Read the model definition and answer for the solid it produces. Units are mm, in the model's axes. Coordinates: 2 decimals unless noted, no trailing zeros. Write each loop counter-clockwise with the first axis right and the second up, starting at its lowest first coordinate (ties: lowest second). Pieces come first, ordered by that corner, then holes. Notation, with made-up numbers: (-30, -32.75) -> (-4, -32.75) arc R25 ccw to (-4, -11.75) -> close; hole circle Ø9 at (67, -2.5). An arc over 180 degrees is marked (long way). One line per item, written item: value. Start each with the question number.
1. Consider line 1 along Z through (x, y) = (-2, 25) (3 decimals); line 2 along Z through (x, y) = (20, 25); line 3 along Y through (x, z) = (-1, 2.4). Determine where each line is inside the solid, lowest interval first.
2. For a pull along Z with two mould halves and no side action, classify faces 1 (the cylindrical face through (-3.451, 22.854, 3.176)), 2 (the cylindrical face through (-3.451, 24.192, 2.165)), 3 (the flat face through (0, 25, 3)), 4 (the flat face through (0, 19, 2)) as pulls with the +Z half, pulls with the -Z half, needs draft (parallel to the pull), parting line crosses it, or undercut.
3. Given P1, Ø2, axis at x = 22, y = 34, coming from the -Z side, flat-ended and moving along its own axis, determine where the tip first touches the part or whether it passes through.
4. Find section A-A, the plane y = 47. Write down the section's boundary in (x, z).
5. Find section B-B, the plane x = -3. Write down the section's boundary in (y, z) (3 decimals).
```python
from build123d import *

# Parameters (mm, degrees)
F0_W     = 50
F0_H     = 50
F1_DEPTH = 5
F2_R     = 0.25
F3_DEPTH = 55.8
F4_R     = 2.25
F4_R_2   = 0.875
F5_DEPTH = 7


with BuildPart() as f1:
    # F0 (on Top) → F1 (new body)
    with BuildSketch(Plane.XY):
        with Locations((25, 25)):
            Rectangle(F0_W, F0_H)
    extrude(amount=F1_DEPTH)

    # F2 (on face) → F3 (cut)
    with BuildSketch(Plane.YZ.offset(50)):
        with Locations((25, 2.5)):
            Circle(F2_R)
    extrude(amount=-F3_DEPTH, mode=Mode.SUBTRACT)

    # F4 (on face) → F5 (join)
    with BuildSketch(Plane(origin=(0, 0, 0), x_dir=(0, -1, 0), z_dir=(-1, 0, 0))):
        with Locations((-25, 2.5)):
            Circle(F4_R)
        with Locations((-25, 2.5)):
            Circle(F4_R_2, mode=Mode.SUBTRACT)
    extrude(amount=F5_DEPTH)


solid = f1.part
```
Answer block:
1. line 1: z = 0.25 to 1.625, 3.375 to 4.75
1. line 2: z = 0 to 2.25, 2.75 to 5
1. line 3: y = 22.75 to 24.13, 25.87 to 27.25
2. face 1: parting line crosses it
2. face 2: undercut
2. face 3: undercut
2. face 4: needs draft
3. P1: stops at z = 0
4. outline: (0, 0) -> (50, 0) -> (50, 5) -> (0, 5) -> close
5. outline: circle Ø4.5 at (25, 2.5); hole circle Ø1.75 at (25, 2.5)
